```python
from build123d import *

# Parameters (mm, degrees)
CROQUIS1_R              = 1
CROQUIS1_W              = 12.5984
CROQUIS1_H              = 22.5298
SALIENTE_EXTRUIR1_DEPTH = 4


with BuildPart() as part:
    # Croquis1 → Saliente-Extruir1 (new body)
    with BuildSketch(Plane(origin=(0, 0, 0), x_dir=(1, 0, 0), z_dir=(0, 1, 0))):
        Polygon((-6.5, -11.2141), (-6.2992, -11.2141), (6.5, -11.2141), (6.5, -8.2141), (11.5, -8.2141), (11.5, -7.5343), (15.5, -7.5343), (15.5, 17.4657), (11.5, 17.4657), (11.5, 21.1455), (-11.5, 21.1455), (-11.5, 17.4657), (-15.5, 17.4657), (-15.5, -7.5343), (-11.5, -7.5343), (-11.5, -8.2141), (-6.5, -8.2141), align=None)
        with Locations((0, -9.036)):
            Circle(CROQUIS1_R, mode=Mode.SUBTRACT)
        with Locations((0, 4.9657)):
            Rectangle(CROQUIS1_W, CROQUIS1_H, mode=Mode.SUBTRACT)
        with Locations((0, 18.9674)):
            Circle(CROQUIS1_R, mode=Mode.SUBTRACT)
    extrude(amount=SALIENTE_EXTRUIR1_DEPTH)


solid = part.part
```
Can you work these out from the model? Positions are in its coordinate system, mm. A direction names the side the tool comes from. Round coordinates to 2 decimals unless told otherwise and drop trailing zeros. Loops run counter-clockwise (first coordinate to the right, second up) from the corner with the lowest first, then second, coordinate; pieces in that order, holes last. Notation, with made-up numbers: M 5,-15.5 L 41,-15.5 A19 ccw 41,0.5 Z; hole C -24,24 d1. An arc over 180 degrees is marked long. Write item = value, one per line. Start each with the question number.
(1) Suppose I cut it at B-B on x = 0. Write out the boundary of the cut face in (y, z).
(2) I need wall thicknesses on line 1 along Z through (x, y) = (0, 1.55); line 2 along X through (y, z) = (0.5, -5); line 3 along Z through (x, y) = (2.5, 0.3). Which ranges of each line are inside material? Lowest first, please.
(3) Suppose I cut it at A-A on z = 4.5. Write out the boundary of the cut face in (x, y).
(4) I'm going to push flat-ended pins straight in: P1, Ø0.9, axis at y = 3, z = 10.5, coming from the -X side; P2, Ø1.1, axis at y = 1.5, z = -20, coming from the -X side; P3, Ø2, axis at x = -8, y = 2.5, coming from the +Z side. Where does each tip first touch, or does it pass through?
(5) If we mould it in two halves opening along Z, with no side actions, what happens to faces 1 (the face through (-14, 2, 7.534)), 2 (the face through (-0.22, 1.97, 10.01)), 3 (the face through (15.5, 2, -5))? For each: released by +Z, released by -Z, zero draft, split by the parting line, or undercut.
(6) Which directions (+Z, -Z, +X, -X, +Y, -Y) give clear straight access to the entire face, cutting with the end or side of a thin tool? Please do faces 4 (the face through (-13, 2, -17.466)), 5 (the face through (14, 2, -17.466)), 6 (the face through (0, 2, 6.299)).
(7) Suppose I cut it at D-D on x = 8. Write out the boundary of the cut face in (y, z), plus the area to 3 significant figures.
(8) Suppose I cut it at C-C on y = 2.65. Write out the boundary of the cut face in (x, z), plus the area to 3 significant figures.
Answer block:
q1.outline = M 0,-21.15 L 4,-21.15 L 4,-19.97 L 0,-19.97 Z; M 0,-17.97 L 4,-17.97 L 4,-16.23 L 0,-16.23 Z; M 0,6.3 L 4,6.3 L 4,8.04 L 0,8.04 Z; M 0,10.04 L 4,10.04 L 4,11.21 L 0,11.21 Z
q2.line_1 = -21.15 to -19.97, -17.97 to -16.23, 6.3 to 8.04, 10.04 to 11.21
q2.line_2 = -15.5 to -6.3, 6.3 to 15.5
q2.line_3 = -21.15 to -16.23, 6.3 to 11.21
q3.outline = M -15.5,0 L -6.3,0 L -6.3,4 L -15.5,4 Z; M 6.3,0 L 15.5,0 L 15.5,4 L 6.3,4 Z
q4.P1 = -6.5
q4.P2 = -11.5
q4.P3 = 8.21
q5.face_1 = released by +Z
q5.face_2 = undercut
q5.face_3 = zero draft
q6.face_4 = -Z, -X, +Y, -Y
q6.face_5 = -Z, +X, +Y, -Y
q6.face_6 = +Y, -Y
q7.outline = M 0,-21.15 L 4,-21.15 L 4,8.21 L 0,8.21 Z
q7.area = 117 mm²
q8.outline = M -15.5,-17.47 L -11.5,-17.47 L -11.5,-21.15 L 11.5,-21.15 L 11.5,-17.47 L 15.5,-17.47 L 15.5,7.53 L 11.5,7.53 L 11.5,8.21 L 6.5,8.21 L 6.5,11.21 L -6.5,11.21 L -6.5,8.21 L -11.5,8.21 L -11.5,7.53 L -15.5,7.53 Z; hole M -6.3,-16.23 L 6.3,-16.23 L 6.3,6.3 L -6.3,6.3 Z; hole C 0,-18.97 d2; hole C 0,9.04 d2
q8.area = 624 mm²
